CAD build for the part. Positions are in the model's coordinates, mm. Face numbers are marked on the shaded views. A direction names the side the tool comes from. Give positions to 0.01 mm unless a question says otherwise; leave off trailing zeros. Loops run counter-clockwise (first coordinate to the right, second up) from the corner with the lowest first, then second, coordinate; pieces in that order, holes last.
```python
from build123d import *

# Parameters (mm, degrees)
F1_DEPTH = 38.1
F2_W     = 73.152
F2_H     = 1.524
F3_DEPTH = 13.97
F4_R     = 4.445
F5_DEPTH = 76.2
F6_R     = 33.655
F6_R_2   = 4.445
F7_DEPTH = 15.24
F8_R     = 2.54
F9_R     = 1.26999


# Not quite as in the source:
# - a fillet or chamfer is up to 0.001 mm smaller than in the source, because OpenCascade refuses the exact size


with BuildPart() as f1:
    # F0 (on Front) → F1 (new body, symmetric)
    with BuildSketch(Plane.XZ):
        Polygon((-36.576, 6.985), (-36.576, -6.985), (36.576, -6.985), (36.576, 6.985), (1.27, 42.291), (1.27, 56.261), (0, 56.261), (-1.27, 56.261), (-1.27, 42.291), align=None)
    extrude(amount=F1_DEPTH, both=True)

    # F2 (on face) → F3 (cut)
    with BuildSketch(Plane(origin=(0, 0, -6.985), x_dir=(1, 0, 0), z_dir=(0, 0, -1))):
        with Locations((0, 37.338)):
            Rectangle(F2_W, F2_H)
        with Locations((0, -37.338)):
            Rectangle(F2_W, F2_H)
    extrude(amount=-F3_DEPTH, mode=Mode.SUBTRACT)

    # F4 (on face) → F5 (cut)
    with BuildSketch(Plane(origin=(0, 0, -6.985), x_dir=(1, 0, 0), z_dir=(0, 0, -1))):
        with Locations((-12.7, 0)):
            Circle(F4_R)
    extrude(amount=-F5_DEPTH, mode=Mode.SUBTRACT)

    # F6 (on face) → F7 (cut)
    with BuildSketch(Plane(origin=(0, 0, -6.985), x_dir=(1, 0, 0), z_dir=(0, 0, -1))):
        Circle(F6_R)
        with Locations((-12.7, 0)):
            Circle(F6_R_2, mode=Mode.SUBTRACT)
    extrude(amount=-F7_DEPTH, mode=Mode.SUBTRACT)

    # F8
    f8_edges = [f1.edges().sort_by_distance(p)[0] for p in [
        (-1.27, 0, 42.291),
        (1.27, 0, 42.291),
    ]]
    fillet(f8_edges, radius=F8_R)

    # F9 (radius 1.27 in the source; OpenCascade refuses exactly that, so slightly less here)
    f9_edges = [f1.edges().sort_by_distance(p)[0] for p in [
        (-1.27, 0, 56.261),
        (0, -38.1, 56.261),
        (1.27, 0, 56.261),
        (0, 38.1, 56.261),
        (-1.27, -38.1, 49.802051),
        (19.294974, -38.1, 24.266026),
        (1.27, -38.1, 49.802051),
        (-1.27, 38.1, 49.802051),
        (1.27, 38.1, 49.802051),
    ]]
    fillet(f9_edges, radius=F9_R)


solid = f1.part
```
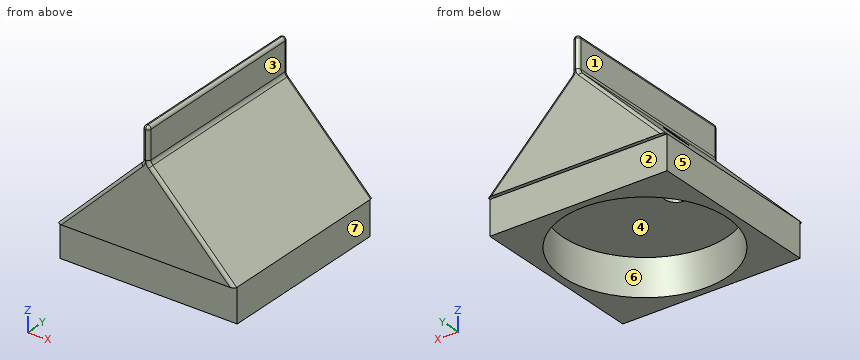
1. Saw through at B-B, the plane z = -1. List the corners of the cut face in (x, y) (3 decimals).
Responses:
outline: (-36.576, -36.576) - (36.576, -36.576) - (36.576, 36.576) - (-36.576, 36.576) - close; hole circle Ø67.31 at (0, 0)
2. Probe line 1 along Y through (x, z) = (0, 4.5) (3 decimals); line 2 along X through (y, z) = (26, 49.5). List the from-to ranges inside material, lowest first.
Responses:
line 1: y = -36.576 to -33.655, 33.655 to 36.576
line 2: x = -1.27 to 1.27
3. Drop flat-ended pins along their axis: pin 1 (1.2 mm diameter, centred on x = -1, y = 37.5, fed in from -Z) (3 decimals); pin 2 (10 mm diameter, centred on x = -9, y = -10.5, fed in from -Z) (3 decimals); pin 3 (2 mm diameter, centred on y = -19.5, z = 43.5, fed in from +X); pin 4 (6 mm diameter, centred on x = -14, z = 37.5, fed in from +Y) (3 decimals). Give the stop position or say it passes through.
Responses:
pin 1: stops at z = 6.985
pin 2: stops at z = 8.255
pin 3: stops at x = 1.41
pin 4: passes through
4. Pull direction X, two halves, no side cores. Call the marked faces 5, 6 and 7: released by +X, released by -X, zero draft, split by the parting line, or undercut.
Responses:
face 5: released by -X
face 6: undercut
face 7: released by +X
5. Tool access for the marked faces 1, 2, 3 and 4: list every direction of +Z, -Z, +X, -X, +Y, -Y with a clear straight run to the whole face (end or side of a thin tool).
Responses:
face 1: +Z, -X, +Y, -Y
face 2: -Z, +X, -X, +Y
face 3: +Z, +X, +Y, -Y
face 4: -Z
